For this review, take the finished solid that the model builds, in its own axes (mm). A direction names the side the tool comes from. Give positions to 0.01 mm unless a question says otherwise; leave off trailing zeros. Write each loop counter-clockwise with the first axis right and the second up, starting at its lowest first coordinate (ties: lowest second). Pieces come first, ordered by that corner, then holes. Notation, with made-up numbers: (21.25, -13.5) -> (31.25, -13.5) arc R13 ccw to (31.25, 0.5) -> close; hole circle Ø9 at (30.25, -34). An arc over 180 degrees is marked (long way). Return JSON: item names as keys, results as strings.
from build123d import *

# Parameters (mm, degrees)
SKETCH1_W           = 22.5
SKETCH1_H           = 45
BOSS_EXTRUDE1_DEPTH = 2.5
SKETCH2_W           = 27.5
SKETCH2_H           = 22.5
BOSS_EXTRUDE2_DEPTH = 2.5
SKETCH3_W           = 27.5
SKETCH3_H           = 22.5
BOSS_EXTRUDE3_DEPTH = 2.5
SKETCH4_W           = 22.5
SKETCH4_H           = 50
BOSS_EXTRUDE4_DEPTH = 2.5
SKETCH5_R           = 1.6
CUT_EXTRUDE1_DEPTH  = 30
FILLET2_R           = 1
FILLET3_R           = 1


with BuildPart() as part:
    # Sketch1 → Boss-Extrude1 (new body)
    with BuildSketch(Plane(origin=(0, 0, 0), x_dir=(0, 0, -1), z_dir=(1, 0, 0))):
        Rectangle(SKETCH1_W, SKETCH1_H)
    extrude(amount=BOSS_EXTRUDE1_DEPTH)

    # Sketch2 → Boss-Extrude2 (add)
    with BuildSketch(Plane(origin=(0, -22.5, 0), x_dir=(-1, 0, 0), z_dir=(0, -1, 0))):
        with Locations((11.25, 0)):
            Rectangle(SKETCH2_W, SKETCH2_H)
    extrude(amount=BOSS_EXTRUDE2_DEPTH)

    # Sketch3 → Boss-Extrude3 (add)
    with BuildSketch(Plane(origin=(0, 22.5, 0), x_dir=(1, 0, 0), z_dir=(0, 1, 0))):
        with Locations((-11.25, 0)):
            Rectangle(SKETCH3_W, SKETCH3_H)
    extrude(amount=BOSS_EXTRUDE3_DEPTH)

    # Sketch4 → Boss-Extrude4 (add)
    with BuildSketch(Plane.ZY.offset(25)):
        Rectangle(SKETCH4_W, SKETCH4_H)
    extrude(amount=BOSS_EXTRUDE4_DEPTH)

    # Sketch5 → Cut-Extrude1 (cut)
    with BuildSketch(Plane.ZY.offset(27.5)):
        Circle(SKETCH5_R)
    extrude(amount=-CUT_EXTRUDE1_DEPTH, mode=Mode.SUBTRACT)

    # Fillet2
    fillet2_edges = [part.edges().sort_by_distance(p)[0] for p in [
        (2.5, 25, 0),
        (-27.5, 25, 0),
    ]]
    fillet(fillet2_edges, radius=FILLET2_R)

    # Fillet3
    fillet3_edges = [part.edges().sort_by_distance(p)[0] for p in [
        (2.5, -25, 0),
        (-27.5, -25, 0),
    ]]
    fillet(fillet3_edges, radius=FILLET3_R)


solid = part.part
1. Add section C-C, the plane z = 0. State the section outline as (x, y) points, plus the area to 3 significant figures.
Results found:
{"outline": "(-27.5, -24) arc R1 ccw to (-26.5, -25) -> (1.5, -25) arc R1 ccw to (2.5, -24) -> (2.5, -1.6) -> (0, -1.6) -> (0, -22.5) -> (-25, -22.5) -> (-25, -1.6) -> (-27.5, -1.6) -> close; (-27.5, 1.6) -> (-25, 1.6) -> (-25, 22.5) -> (0, 22.5) -> (0, 1.6) -> (2.5, 1.6) -> (2.5, 24) arc R1 ccw to (1.5, 25) -> (-26.5, 25) arc R1 ccw to (-27.5, 24) -> close", "area": "358 mm²"}
2. The part is to be moulded in two halves that separate along X. For faces 1 (the cylindrical face through (1.23, -0.97, -1.27)), 2 (the cylindrical face through (-27.215, -24.699, 0.158)), 3 (the flat face through (-25, 0, 2)), say which applies: +X half, -X half, draft (parallel to the pull), parting line (faces both ways), or undercut.
Results found:
{"face 1": "draft", "face 2": "-X half", "face 3": "undercut"}
3. Add section B-B, the plane x = -7. State the section outline as (y, z) points.
Results found:
{"outline": "(-25, -11.25) -> (-22.5, -11.25) -> (-22.5, 11.25) -> (-25, 11.25) -> close; (22.5, -11.25) -> (25, -11.25) -> (25, 11.25) -> (22.5, 11.25) -> close"}
4. For pin 1 (2.5 mm diameter, centred on y = 0, z = 0, fed in from +X), flat-tipped, find the tip position at first contact; note if it passes through.
Results found:
{"pin 1": "passes through"}
5. To check wall thickness, follow probe 1 along Y at (x, z) = (-23.5, 0); probe 2 along X at (y, z) = (16.5, 1); probe 3 along Y at (x, z) = (-25.8, 0). State the ranges of each line that lie inside material, in increasing order.
Results found:
{"probe 1": "y = -25 to -22.5, 22.5 to 25", "probe 2": "x = -27.5 to -25, 0 to 2.5", "probe 3": "y = -25 to -1.6, 1.6 to 25"}
6. For faces 4 (the flat face through (0, 0, -2)), 5 (the flat face through (-12, -25, 0)), list the 3-axis set-ups (+Z, -Z, +X, -X, +Y, -Y) from which the entire face can be reached by the end or side of a thin tool; tool diameter is ignored.
Results found:
{"face 4": "+Z, -Z", "face 5": "+Z, -Z, +X, -X, -Y"}
7. Add section A-A, the plane y = -20.5. State the section outline as (x, z) points.
Results found:
{"outline": "(-27.5, -11.25) -> (-25, -11.25) -> (-25, 11.25) -> (-27.5, 11.25) -> close; (0, -11.25) -> (2.5, -11.25) -> (2.5, 11.25) -> (0, 11.25) -> close"}
8. Add section D-D, the plane y = 0. State the section outline as (x, z) points.
Results found:
{"outline": "(-27.5, -11.25) -> (-25, -11.25) -> (-25, -1.6) -> (-27.5, -1.6) -> close; (-27.5, 1.6) -> (-25, 1.6) -> (-25, 11.25) -> (-27.5, 11.25) -> close; (0, -11.25) -> (2.5, -11.25) -> (2.5, -1.6) -> (0, -1.6) -> close; (0, 1.6) -> (2.5, 1.6) -> (2.5, 11.25) -> (0, 11.25) -> close"}
